Design review of the part built by this model. Coordinates are the model's own, in mm. Coordinates: 2 decimals unless noted, no trailing zeros. Loops run counter-clockwise (first coordinate to the right, second up) from the corner with the lowest first, then second, coordinate; pieces in that order, holes last. Notation, with made-up numbers: M 43,75.25 L 87,75.25 A38 cw 87,114.25 Z; hole C -18.75,61.25 d2. An arc over 180 degrees is marked long. Answer as a JSON object with one key per item and string values. Group by question number.
1. Consider section B-B (x = 0). State the section outline as (y, z) points.
2. Consider section A-A (z = 0). State the section outline as (x, y) points, then the cut area to 3 significant figures.
3. Consider section D-D (z = -38). State the section outline as (x, y) points, then the cut area to 3 significant figures.
4. To check wall thickness, follow probe 1 along Z at (x, y) = (-27, 2.5); probe 2 along X at (y, z) = (3, -11); probe 3 along Z at (x, y) = (85, -2.5). State the ranges of each line that lie inside material, in increasing order.
5. Consider section C-C (y = 0.5). Count the separate pieces of the cut face and the enclosed holes in it, then the cut area to 3 significant figures.
6. Insertion check: pin 1 (5 mm diameter, centred on x = 44.9, z = 44.9, fed in from +Y); pin 2 (1 mm diameter, centred on x = 76.5, y = -3.5, fed in from -Z). Each pin has a flat end and moves straight along its axis. Give the tip position at first contact, or say it passes through.
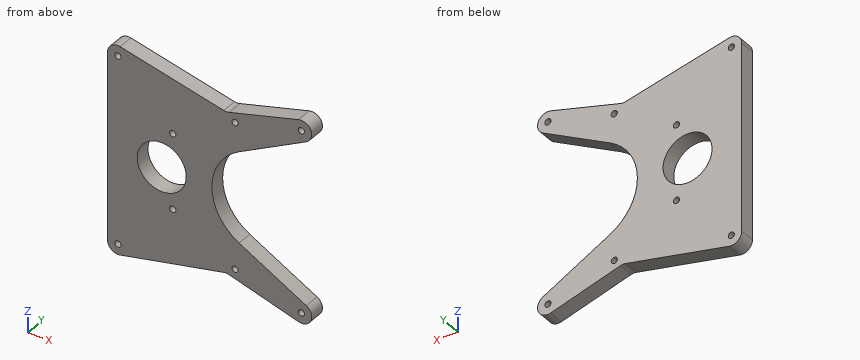
from build123d import *

# Parameters (mm, degrees)
SKETCH2_R           = 1.905
SKETCH2_R_2         = 15.012499947
BOSS_EXTRUDE1_DEPTH = 4.7625


with BuildPart() as part:
    # Sketch2 → Boss-Extrude1 (new body, symmetric)
    with BuildSketch(Plane(origin=(0, 0, 0), x_dir=(1, 0, 0), z_dir=(0, 1, 0))):
        with BuildLine():
            Line((47.431459746, 27.946405755), (88.599086108, 50.143751648))
            ThreePointArc((88.599086108, 50.143751648), (91.466763895, 58.127150721), (83.838709673, 61.83808395))
            Line((83.838709673, 61.83808395), (41.161290327, 49.627981648))
            ThreePointArc((41.161290327, 49.627981648), (39.600064271, 49.38574116), (38.027358671, 49.536420772))
            Line((38.027358671, 49.536420772), (-25.448996349, 63.747156504))
            ThreePointArc((-25.448996349, 63.747156504), (-30.805729247, 62.50693539), (-33.186259621, 57.550544477))
            Line((-33.186259621, 57.550544477), (-33.186259621, -57.550544477))
            ThreePointArc((-33.186259621, -57.550544477), (-30.805729247, -62.50693539), (-25.448996349, -63.747156504))
            Line((-25.448996349, -63.747156504), (38.027358671, -49.536420772))
            ThreePointArc((38.027358671, -49.536420772), (39.600064271, -49.38574116), (41.161290327, -49.627981648))
            Line((41.161290327, -49.627981648), (83.838709673, -61.83808395))
            ThreePointArc((83.838709673, -61.83808395), (91.466763895, -58.127150721), (88.599086108, -50.143751648))
            Line((88.599086108, -50.143751648), (47.431459746, -27.946405755))
            ThreePointArc((47.431459746, -27.946405755), (30.75, 0), (47.431459746, 27.946405755))
        make_face()
        with Locations((6.766967201, -23.085378057)):
            Circle(SKETCH2_R, mode=Mode.SUBTRACT)
        with Locations((44.901280605, -44.901280605)):
            Circle(SKETCH2_R, mode=Mode.SUBTRACT)
        Circle(SKETCH2_R_2, mode=Mode.SUBTRACT)
        with Locations((6.766967201, 23.085378057)):
            Circle(SKETCH2_R, mode=Mode.SUBTRACT)
        with Locations((44.901280605, 44.901280605)):
            Circle(SKETCH2_R, mode=Mode.SUBTRACT)
        with Locations((85.585378057, 55.733032799)):
            Circle(SKETCH2_R, mode=Mode.SUBTRACT)
        with Locations((-26.836259621, 57.550544477)):
            Circle(SKETCH2_R, mode=Mode.SUBTRACT)
        with Locations((85.585378057, -55.733032799)):
            Circle(SKETCH2_R, mode=Mode.SUBTRACT)
        with Locations((-26.836259621, -57.550544477)):
            Circle(SKETCH2_R, mode=Mode.SUBTRACT)
    extrude(amount=BOSS_EXTRUDE1_DEPTH, both=True)


solid = part.part
Findings below:
{
 "1": {"outline": "M -4.76,-58.05 L 4.76,-58.05 L 4.76,-15.01 L -4.76,-15.01 Z; M -4.76,15.01 L 4.76,15.01 L 4.76,58.05 L -4.76,58.05 Z"},
 "2": {"outline": "M -33.19,-4.76 L -15.01,-4.76 L -15.01,4.76 L -33.19,4.76 Z; M 15.01,-4.76 L 30.75,-4.76 L 30.75,4.76 L 15.01,4.76 Z", "area": "323 mm^2"},
 "3": {"outline": "M -33.19,-4.76 L 66.08,-4.76 L 66.08,4.76 L -33.19,4.76 Z", "area": "945 mm^2"},
 "4": {"probe 1": "z = -63.9 to -59.45, -55.65 to 55.65, 59.45 to 63.9", "probe 2": "x = -33.19 to -10.22, 10.22 to 32.72", "probe 3": "z = -62.06 to -57.55, -53.92 to -48.2, 48.2 to 53.92, 57.55 to 62.06"},
 "5": {"separate pieces": "1", "enclosed holes": "9", "area": "9,190 mm^2"},
 "6": {"pin 1": "stops at y = 4.76", "pin 2": "stops at z = -59.88"}
}
